from build123d import *

# Parameters (mm, degrees)
ISO_START                                 = 2.649023341
ISO_SPUR_GEAR_1_5M_20T_20PA_3FW_2_R       = 0.4
ISO_SPUR_GEAR_1_5M_20T_20PA_3FW_S20_DEPTH = 3
BOSS_EXTRUDE1_DEPTH                       = 4
BOSS_EXTRUDE1_DEPTH_BACK                  = 3
SKETCH1_R                                 = 3
SKETCH2_R                                 = 2.4
CUT_EXTRUDE1_DEPTH                        = 3.2


# Read off the part's stored shape, not the designer's step: ISO - Spur gear 1.5M 20T 20PA 3FW ---S20A75H50L0.8N
with BuildPart() as part:
    # ISO - Spur gear 1.5M 20T 20PA 3FW -- 2 → ISO - Spur gear 1.5M 20T 20PA 3FW ---S20 (new body)
    with BuildSketch(Plane.YZ.offset(ISO_START)):
        with BuildLine():
            ThreePointArc((-13.663753379, 26.133903668), (-14.053655616, 26.200458221), (-14.445041168, 26.257647498))
            ThreePointArc((-14.445041168, 26.257647498), (-15.414573535, 24.741730478), (-15.891009909, 23.006505477))
            ThreePointArc((-15.891009909, 23.006505477), (-16.634824289, 23.027600602), (-17.37863867, 23.006505477))
            ThreePointArc((-17.37863867, 23.006505477), (-17.855075045, 24.741730477), (-18.824607411, 26.257647498))
            ThreePointArc((-18.824607411, 26.257647498), (-19.215992963, 26.200458221), (-19.6058952, 26.133903668))
            ThreePointArc((-19.6058952, 26.133903668), (-20.059531154, 24.39257893), (-19.976435058, 22.59505495))
            ThreePointArc((-19.976435058, 22.59505495), (-20.690363323, 22.385266321), (-21.391254085, 22.135352381))
            ThreePointArc((-21.391254085, 22.135352381), (-22.380586018, 23.638422489), (-23.771110214, 24.780543271))
            ThreePointArc((-23.771110214, 24.780543271), (-24.125667535, 24.605208251), (-24.475920111, 24.421424692))
            ThreePointArc((-24.475920111, 24.421424692), (-24.369254604, 22.625145234), (-23.734760063, 20.941276444))
            ThreePointArc((-23.734760063, 20.941276444), (-24.348917941, 20.521139636), (-24.938277012, 20.066870198))
            ThreePointArc((-24.938277012, 20.066870198), (-26.343661801, 21.190654438), (-28.01906363, 21.847180243))
            ThreePointArc((-28.01906363, 21.847180243), (-28.302086179, 21.570862491), (-28.578403931, 21.287839942))
            ThreePointArc((-28.578403931, 21.287839942), (-27.921878126, 19.612438113), (-26.798093886, 18.207053324))
            ThreePointArc((-26.798093886, 18.207053324), (-27.252363324, 17.617694253), (-27.672500133, 17.003536375))
            ThreePointArc((-27.672500133, 17.003536375), (-29.356368922, 17.638030916), (-31.15264838, 17.744696423))
            ThreePointArc((-31.15264838, 17.744696423), (-31.336431939, 17.394443847), (-31.511766959, 17.039886526))
            ThreePointArc((-31.511766959, 17.039886526), (-30.369646177, 15.64936233), (-28.866576069, 14.660030397))
            ThreePointArc((-28.866576069, 14.660030397), (-29.116490009, 13.959139635), (-29.326278638, 13.24521137))
            ThreePointArc((-29.326278638, 13.24521137), (-31.123802618, 13.328307466), (-32.865127356, 12.874671512))
            ThreePointArc((-32.865127356, 12.874671512), (-32.931681909, 12.484769275), (-32.988871186, 12.093383723))
            ThreePointArc((-32.988871186, 12.093383723), (-31.472954165, 11.123851357), (-29.737729165, 10.647414982))
            ThreePointArc((-29.737729165, 10.647414982), (-29.75882429, 9.903600602), (-29.737729165, 9.159786221))
            ThreePointArc((-29.737729165, 9.159786221), (-31.472954166, 8.683349847), (-32.988871186, 7.71381748))
            ThreePointArc((-32.988871186, 7.71381748), (-32.931681909, 7.322431928), (-32.865127356, 6.932529691))
            ThreePointArc((-32.865127356, 6.932529691), (-31.123802618, 6.478893737), (-29.326278638, 6.561989833))
            ThreePointArc((-29.326278638, 6.561989833), (-29.116490009, 5.848061568), (-28.866576069, 5.147170806))
            ThreePointArc((-28.866576069, 5.147170806), (-30.369646177, 4.157838873), (-31.511766959, 2.767314677))
            ThreePointArc((-31.511766959, 2.767314677), (-31.336431939, 2.412757356), (-31.15264838, 2.06250478))
            ThreePointArc((-31.15264838, 2.06250478), (-29.356368922, 2.169170287), (-27.672500133, 2.803664828))
            ThreePointArc((-27.672500133, 2.803664828), (-27.252363324, 2.18950695), (-26.798093886, 1.600147879))
            ThreePointArc((-26.798093886, 1.600147879), (-27.921878126, 0.19476309), (-28.578403931, -1.480638739))
            ThreePointArc((-28.578403931, -1.480638739), (-28.302086179, -1.763661288), (-28.01906363, -2.03997904))
            ThreePointArc((-28.01906363, -2.03997904), (-26.343661801, -1.383453235), (-24.938277012, -0.259668995))
            ThreePointArc((-24.938277012, -0.259668995), (-24.348917941, -0.713938433), (-23.734760063, -1.134075241))
            ThreePointArc((-23.734760063, -1.134075241), (-24.369254604, -2.817944031), (-24.475920111, -4.614223489))
            ThreePointArc((-24.475920111, -4.614223489), (-24.125667535, -4.798007048), (-23.771110214, -4.973342068))
            ThreePointArc((-23.771110214, -4.973342068), (-22.380586018, -3.831221286), (-21.391254085, -2.328151178))
            ThreePointArc((-21.391254085, -2.328151178), (-20.690363323, -2.578065118), (-19.976435058, -2.787853747))
            ThreePointArc((-19.976435058, -2.787853747), (-20.059531154, -4.585377727), (-19.6058952, -6.326702465))
            ThreePointArc((-19.6058952, -6.326702465), (-19.215992963, -6.393257018), (-18.824607411, -6.450446295))
            ThreePointArc((-18.824607411, -6.450446295), (-17.855075045, -4.934529274), (-17.37863867, -3.199304274))
            ThreePointArc((-17.37863867, -3.199304274), (-16.634824289, -3.220399398), (-15.891009909, -3.199304274))
            ThreePointArc((-15.891009909, -3.199304274), (-15.414573535, -4.934529275), (-14.445041168, -6.450446295))
            ThreePointArc((-14.445041168, -6.450446295), (-14.053655616, -6.393257018), (-13.663753379, -6.326702465))
            ThreePointArc((-13.663753379, -6.326702465), (-13.210117425, -4.585377727), (-13.293213521, -2.787853747))
            ThreePointArc((-13.293213521, -2.787853747), (-12.579285256, -2.578065118), (-11.878394494, -2.328151178))
            ThreePointArc((-11.878394494, -2.328151178), (-10.889062561, -3.831221286), (-9.498538365, -4.973342068))
            ThreePointArc((-9.498538365, -4.973342068), (-9.143981044, -4.798007048), (-8.793728468, -4.614223489))
            ThreePointArc((-8.793728468, -4.614223489), (-8.900393975, -2.817944031), (-9.534888516, -1.134075241))
            ThreePointArc((-9.534888516, -1.134075241), (-8.920730638, -0.713938433), (-8.331371567, -0.259668995))
            ThreePointArc((-8.331371567, -0.259668995), (-6.925986778, -1.383453235), (-5.250584949, -2.03997904))
            ThreePointArc((-5.250584949, -2.03997904), (-4.9675624, -1.763661288), (-4.691244648, -1.480638739))
            ThreePointArc((-4.691244648, -1.480638739), (-5.347770453, 0.19476309), (-6.471554693, 1.600147879))
            ThreePointArc((-6.471554693, 1.600147879), (-6.017285255, 2.18950695), (-5.597148447, 2.803664828))
            ThreePointArc((-5.597148447, 2.803664828), (-3.913279657, 2.169170287), (-2.117000199, 2.06250478))
            ThreePointArc((-2.117000199, 2.06250478), (-1.93321664, 2.412757356), (-1.75788162, 2.767314677))
            ThreePointArc((-1.75788162, 2.767314677), (-2.900002402, 4.157838873), (-4.40307251, 5.147170806))
            ThreePointArc((-4.40307251, 5.147170806), (-4.15315857, 5.848061568), (-3.943369941, 6.561989833))
            ThreePointArc((-3.943369941, 6.561989833), (-2.145845961, 6.478893737), (-0.404521223, 6.932529691))
            ThreePointArc((-0.404521223, 6.932529691), (-0.33796667, 7.322431928), (-0.280777393, 7.71381748))
            ThreePointArc((-0.280777393, 7.71381748), (-1.796694413, 8.683349847), (-3.531919414, 9.159786221))
            ThreePointArc((-3.531919414, 9.159786221), (-3.51082429, 9.903600601), (-3.531919414, 10.647414982))
            ThreePointArc((-3.531919414, 10.647414982), (-1.796694414, 11.123851357), (-0.280777393, 12.093383723))
            ThreePointArc((-0.280777393, 12.093383723), (-0.33796667, 12.484769275), (-0.404521223, 12.874671512))
            ThreePointArc((-0.404521223, 12.874671512), (-2.145845961, 13.328307466), (-3.943369941, 13.24521137))
            ThreePointArc((-3.943369941, 13.24521137), (-4.15315857, 13.959139635), (-4.40307251, 14.660030397))
            ThreePointArc((-4.40307251, 14.660030397), (-2.900002402, 15.64936233), (-1.75788162, 17.039886526))
            ThreePointArc((-1.75788162, 17.039886526), (-1.93321664, 17.394443847), (-2.117000199, 17.744696423))
            ThreePointArc((-2.117000199, 17.744696423), (-3.913279657, 17.638030916), (-5.597148447, 17.003536375))
            ThreePointArc((-5.597148447, 17.003536375), (-6.017285255, 17.617694253), (-6.471554693, 18.207053324))
            ThreePointArc((-6.471554693, 18.207053324), (-5.347770453, 19.612438113), (-4.691244648, 21.287839942))
            ThreePointArc((-4.691244648, 21.287839942), (-4.9675624, 21.570862491), (-5.250584949, 21.847180243))
            ThreePointArc((-5.250584949, 21.847180243), (-6.925986778, 21.190654438), (-8.331371567, 20.066870198))
            ThreePointArc((-8.331371567, 20.066870198), (-8.920730638, 20.521139636), (-9.534888516, 20.941276444))
            ThreePointArc((-9.534888516, 20.941276444), (-8.900393975, 22.625145234), (-8.793728468, 24.421424692))
            ThreePointArc((-8.793728468, 24.421424692), (-9.143981044, 24.605208251), (-9.498538365, 24.780543271))
            ThreePointArc((-9.498538365, 24.780543271), (-10.889062561, 23.638422489), (-11.878394494, 22.135352381))
            ThreePointArc((-11.878394494, 22.135352381), (-12.579285256, 22.385266321), (-13.293213521, 22.59505495))
            ThreePointArc((-13.293213521, 22.59505495), (-13.210117425, 24.39257893), (-13.663753379, 26.133903668))
        make_face()
        with Locations((-16.63482429, 9.903600602)):
            Circle(ISO_SPUR_GEAR_1_5M_20T_20PA_3FW_2_R, mode=Mode.SUBTRACT)
    extrude(amount=ISO_SPUR_GEAR_1_5M_20T_20PA_3FW_S20_DEPTH)

    # Sketch1 → Boss-Extrude1 (add, two sides: drawn at the far end of the back side and taken through both)
    with BuildSketch(Plane.ZY.offset(-2.649023341).offset(-BOSS_EXTRUDE1_DEPTH_BACK)):
        with Locations((9.903600602, -16.63482429)):
            Circle(SKETCH1_R)
    extrude(amount=BOSS_EXTRUDE1_DEPTH + BOSS_EXTRUDE1_DEPTH_BACK)

    # Sketch2 → Cut-Extrude1 (cut)
    with BuildSketch(Plane.ZY.offset(1.350976659)):
        with Locations((9.903600602, -16.63482429)):
            Circle(SKETCH2_R)
    extrude(amount=-CUT_EXTRUDE1_DEPTH, mode=Mode.SUBTRACT)


solid = part.part
Check sheet for the modelled part. Datum: model origin and axes. Units: mm. A direction names the side the tool comes from. Round coordinates to 2 decimals unless told otherwise and drop trailing zeros. Loops run counter-clockwise (first coordinate to the right, second up) from the corner with the lowest first, then second, coordinate; pieces in that order, holes last. Notation, with made-up numbers: (17, 69) - (66, 69) arc R11 cw to (66, 83) - close; hole circle Ø2 at (10, 9). An arc over 180 degrees is marked (long way). Answer as CSV lines item,"result". Start each with the question number.
Item 1: Release check for a two-part mould opening along Z. For faces 5 (the cylindrical face through (4.128, -15.404, 24.765)), 6 (the cylindrical face through (4.128, -24.364, -2.793)), 7 (the cylindrical face through (4.13, -26.37, -1.4)) record: +Z half, -Z half, draft (parallel to the pull), parting line (faces both ways), or undercut.
Item 2: Scan lines: line 1 (Y direction, x = 3.75, z = -3.5); line 2 (Z direction, x = 4.75, y = -28); line 3 (X direction, y = -6.5, z = 9.5). Record each from-to range of solid material in increasing order. Write a range as [from, to].
Item 3: Depth check by flat-ended pin: P1, Ø1, axis at y = -13, z = 18.5, coming from the -X side; P2, Ø8, axis at y = -18, z = 7, coming from the -X side; P3, Ø3, axis at x = 4, y = -29, coming from the +Z side. Enter the tip coordinate at first touch or a pass-through.
Item 4: Section check C-C (x = 1). Record the boundary of the cut face in (y, z), and give its area (3 significant figures).
Item 5: Set-up check for faces 1 (the cylindrical face through (4.128, -8.895, -2.843)), 2 (the cylindrical face through (4.128, -17.865, -4.958)), 3 (the cylindrical face through (0.227, -14.255, 9.591)), 4 (the cylindrical face through (4.13, -5.36, 19.59)): record each of +Z, -Z, +X, -X, +Y, -Y from which the full face is reachable in a straight line by a thin tool's end or side.
Item 6: Section check D-D (z = 16). Record the boundary of the cut face in (x, y), and give its area (3 significant figures).
Item 7: Section check A-A (z = 10). Record the boundary of the cut face in (x, y), and give its area (3 significant figures).
Item 8: Section check B-B (y = -15). Record the boundary of the cut face in (x, z).
Report:
1,face 5,"+Z half"
1,face 6,"undercut"
1,face 7,"-Z half"
2,line 1,"y = [-24.47, -22.1], [-20.07, -17.42], [-15.85, -13.2], [-11.17, -8.8]"
2,line 2,"z = [-2.04, 0.06], [2.63, 17.17], [19.75, 21.84]"
2,line 3,"x = [2.65, 5.65]"
3,P1,"stops at x = 2.65"
3,P2,"stops at x = -1.35"
3,P3,"stops at z = 21.85"
4,outline,"circle Ø6 at (-16.63, 9.9); hole circle Ø4.8 at (-16.63, 9.9)"
4,area,"10.2 mm2"
5,face 1,"+X, -X"
5,face 2,"-Z, +X, -X"
5,face 3,"-X"
5,face 4,"+X, -X, +Y"
6,outline,"(2.65, -30.73) - (5.65, -30.73) - (5.65, -2.54) - (2.65, -2.54) - close"
6,area,"84.6 mm2"
7,outline,"(-1.35, -19.63) - (2.65, -19.63) - (2.65, -29.76) - (5.65, -29.76) - (5.65, -3.51) - (2.65, -3.51) - (2.65, -13.64) - (-1.35, -13.64) - (-1.35, -14.24) - (1.85, -14.24) - (1.85, -19.03) - (-1.35, -19.03) - close"
7,area,"87.4 mm2"
8,outline,"(-1.35, 7.39) - (2.65, 7.39) - (2.65, -5.71) - (5.65, -5.71) - (5.65, 25.52) - (2.65, 25.52) - (2.65, 12.42) - (-1.35, 12.42) - (-1.35, 11.66) - (1.85, 11.66) - (1.85, 8.15) - (-1.35, 8.15) - close"
